Build history of the part. All positions in model axes, mm. Face numbers are marked on the shaded views. A direction names the side the tool comes from. Give positions to 0.01 mm unless a question says otherwise; leave off trailing zeros. Order: outer loops, then holes, each group sorted by start corner. A loop starts at its lowest first (then second) coordinate and runs counter-clockwise, first axis right, second up. Notation, with made-up numbers: M 56,74 L 80,74 A25 ccw 80,103 Z; hole C 67.25,21 d10. An arc over 180 degrees is marked long. Answer as CSV lines item,"result".
from build123d import *
from OCP.BRepFilletAPI import BRepFilletAPI_MakeChamfer

# Parameters (mm, degrees)
ODGI_CIE_BAZOWE1_DEPTH     = 200
SZKIC25_W                  = 265
SZKIC25_H                  = 70
WYTNIJ_WYCI_GNI_CIE2_DEPTH = 94
SFAZOWANIE1_SIZE           = 6
SFAZOWANIE1_SIZE2          = 10.392304845
ZAOKR_GLENIE1_R            = 10
OTW_R_POD_RUB_M51_D        = 5.5
OTW_R_POD_RUB_M51_DEPTH    = 3
OTW_R_POD_RUB_M61_D        = 6.6
OTW_R_POD_RUB_M61_DEPTH    = 3
OTW_R_POD_RUB_M52_D        = 5.5
OTW_R_POD_RUB_M62_D        = 6.6
OTW_R_POD_RUB_M62_DEPTH    = 10
OTW_R_POD_RUB_M62_TIP      = 1.982840043
WYTNIJ_WYCI_GNI_CIE3_REACH = 281.957
SZKIC48_R                  = 7
WYTNIJ_WYCI_GNI_CIE4_DEPTH = 10


# Sheet-metal steps are written as plain solids
with BuildPart() as part:
    # Szkic1 → Odgięcie bazowe1 (new, symmetric)
    with BuildSketch(Plane(origin=(0, 0, 0), x_dir=(0, 0, -1), z_dir=(1, 0, 0))):
        with BuildLine():
            Line((-60, 135), (-60, 4))
            ThreePointArc((-60, 4), (-58.828427125, 1.171572875), (-56, 0))
            Line((-56, 0), (56, 0))
            ThreePointArc((56, 0), (58.828427125, 1.171572875), (60, 4))
            Line((60, 4), (60, 150))
            Line((60, 150), (63, 150))
            Line((63, 150), (63, 4))
            ThreePointArc((63, 4), (60.949747468, -0.949747468), (56, -3))
            Line((56, -3), (-56, -3))
            ThreePointArc((-56, -3), (-60.949747468, -0.949747468), (-63, 4))
            Line((-63, 4), (-63, 135))
            Line((-63, 135), (-60, 135))
        make_face()
    extrude(amount=ODGI_CIE_BAZOWE1_DEPTH, both=True)

    # Szkic25 → Wytnij-wyciągnięcie2 (cut)
    with BuildSketch(Plane.XY.offset(63)):
        with Locations((-67.5, 32)):
            Rectangle(SZKIC25_W, SZKIC25_H)
    extrude(amount=-WYTNIJ_WYCI_GNI_CIE2_DEPTH, mode=Mode.SUBTRACT)

    # Sfazowanie1: one chamfer whose edges measure the first distance from different faces: ONE call of the kernel's chamfer builder (chamfer() names one face for all edges)
    sfazowanie1_edges_1 = [part.edges().sort_by_distance(p)[0] for p in [
        (-200, 150, -61.5),
        (-200, -1.5, -31),
    ]]
    sfazowanie1_side_1 = [part.faces().sort_by_distance(p)[0] for p in [
        (-200, -1.436894117, -43.5),
    ]]
    sfazowanie1_edges_2 = [part.edges().sort_by_distance(p)[0] for p in [
        (-200, 135, 61.5),
        (-200, 67, 61.5),
    ]]
    sfazowanie1_side_2 = [part.faces().sort_by_distance(p)[0] for p in [
        (-200, 101, 61.5),
    ]]
    sfazowanie1_edges_3 = [part.edges().sort_by_distance(p)[0] for p in [
        (200, 150, -61.5),
        (200, 135, 61.5),
    ]]
    sfazowanie1_side_3 = [part.faces().sort_by_distance(p)[0] for p in [
        (200, 0.451769567, 59.548230433),
    ]]
    sfazowanie1 = BRepFilletAPI_MakeChamfer(part.part.solid().wrapped)
    for e in sfazowanie1_edges_1:
        sfazowanie1.Add(SFAZOWANIE1_SIZE, SFAZOWANIE1_SIZE2, e.wrapped, sfazowanie1_side_1[0].wrapped)  # the first distance lies on this face
    for e in sfazowanie1_edges_2:
        sfazowanie1.Add(SFAZOWANIE1_SIZE, SFAZOWANIE1_SIZE2, e.wrapped, sfazowanie1_side_2[0].wrapped)  # the first distance lies on this face
    for e in sfazowanie1_edges_3:
        sfazowanie1.Add(SFAZOWANIE1_SIZE, SFAZOWANIE1_SIZE2, e.wrapped, sfazowanie1_side_3[0].wrapped)  # the first distance lies on this face
    add(Compound.cast(sfazowanie1.Shape()), mode=Mode.REPLACE)

    # Zaokrąglenie1
    zaokr_glenie1_edges = [part.edges().sort_by_distance(p)[0] for p in [
        (65, -1.5, -31),
        (65, 67, 61.5),
    ]]
    fillet(zaokr_glenie1_edges, radius=ZAOKR_GLENIE1_R)

    # Otwór pod śrubę M51
    with Locations(Plane.XY.offset(63)):
        with Locations((144, 79), (116, 79), (144, 51), (116, 51), (130, 65)):
            Hole(OTW_R_POD_RUB_M51_D / 2, depth=OTW_R_POD_RUB_M51_DEPTH)

    # Otwór pod śrubę M61
    with Locations(Plane(origin=(0, 0, -63), x_dir=(-1, 0, 0), z_dir=(0, 0, -1))):
        with Locations((-70, 84.5), (-70, 45.5), (50, 84.5), (50, 45.5), (170, 84.5), (170, 45.5)):
            Hole(OTW_R_POD_RUB_M61_D / 2, depth=OTW_R_POD_RUB_M61_DEPTH)

    # Otwór pod śrubę M52 (through all)
    with Locations(Plane(origin=(0, 0, -63), x_dir=(-1, 0, 0), z_dir=(0, 0, -1))):
        with Locations((-172.5, 125), (-57.5, 125), (57.5, 125), (172.5, 125)):
            Hole(OTW_R_POD_RUB_M52_D / 2)

    # Otwór pod śrubę M62
    with Locations(Plane(origin=(0, -3, 0), x_dir=(-1, 0, 0), z_dir=(0, -1, 0))):
        with Locations((-190, 47.25), (-80, 47.25), (-151, 39.85), (-119, 39.85), (-190, -47.25), (-151, -39.85), (-119, -39.85), (-80, -47.25)):
            Hole(OTW_R_POD_RUB_M62_D / 2, depth=OTW_R_POD_RUB_M62_DEPTH)
            with Locations((0, 0, -(OTW_R_POD_RUB_M62_DEPTH + OTW_R_POD_RUB_M62_TIP / 2))):  # 118° drill point
                Cone(0, OTW_R_POD_RUB_M62_D / 2, OTW_R_POD_RUB_M62_TIP, mode=Mode.SUBTRACT)

    # Szkic43 → Wytnij-wyciągnięcie3 (cut, up to next)
    with BuildSketch(Plane(origin=(0, 0, -63), x_dir=(-1, 0, 0), z_dir=(0, 0, -1)), mode=Mode.PRIVATE) as wytnij_wyci_gni_cie3_sk1:
        with BuildLine():
            Line((130, 146), (180, 146))
            ThreePointArc((180, 146), (182, 144), (180, 142))
            Line((180, 142), (130, 142))
            ThreePointArc((130, 142), (128, 144), (130, 146))
        make_face()
    wytnij_wyci_gni_cie3_tool1 = extrude(wytnij_wyci_gni_cie3_sk1.sketch, amount=-WYTNIJ_WYCI_GNI_CIE3_REACH, mode=Mode.PRIVATE) & part.part
    # Szkic43 → Wytnij-wyciągnięcie3 (cut, up to next)
    with BuildSketch(Plane(origin=(0, 0, -63), x_dir=(-1, 0, 0), z_dir=(0, 0, -1)), mode=Mode.PRIVATE) as wytnij_wyci_gni_cie3_sk2:
        with BuildLine():
            Line((70, 146), (120, 146))
            ThreePointArc((120, 146), (122, 144), (120, 142))
            Line((120, 142), (70, 142))
            ThreePointArc((70, 142), (68, 144), (70, 146))
        make_face()
    wytnij_wyci_gni_cie3_tool2 = extrude(wytnij_wyci_gni_cie3_sk2.sketch, amount=-WYTNIJ_WYCI_GNI_CIE3_REACH, mode=Mode.PRIVATE) & part.part
    # Szkic43 → Wytnij-wyciągnięcie3 (cut, up to next)
    with BuildSketch(Plane(origin=(0, 0, -63), x_dir=(-1, 0, 0), z_dir=(0, 0, -1)), mode=Mode.PRIVATE) as wytnij_wyci_gni_cie3_sk3:
        with BuildLine():
            Line((10, 146), (60, 146))
            ThreePointArc((60, 146), (62, 144), (60, 142))
            Line((60, 142), (10, 142))
            ThreePointArc((10, 142), (8, 144), (10, 146))
        make_face()
    wytnij_wyci_gni_cie3_tool3 = extrude(wytnij_wyci_gni_cie3_sk3.sketch, amount=-WYTNIJ_WYCI_GNI_CIE3_REACH, mode=Mode.PRIVATE) & part.part
    add(wytnij_wyci_gni_cie3_tool1.solids().sort_by_distance((-155, 144, -63))[0], mode=Mode.SUBTRACT)
    add(wytnij_wyci_gni_cie3_tool2.solids().sort_by_distance((-95, 144, -63))[0], mode=Mode.SUBTRACT)
    add(wytnij_wyci_gni_cie3_tool3.solids().sort_by_distance((-35, 144, -63))[0], mode=Mode.SUBTRACT)

    # Szkic48 → Wytnij-wyciągnięcie4 (cut)
    with BuildSketch(Plane.XY.offset(63)):
        with Locations((130, 65)):
            Circle(SZKIC48_R)
    extrude(amount=-WYTNIJ_WYCI_GNI_CIE4_DEPTH, mode=Mode.SUBTRACT)


solid = part.part
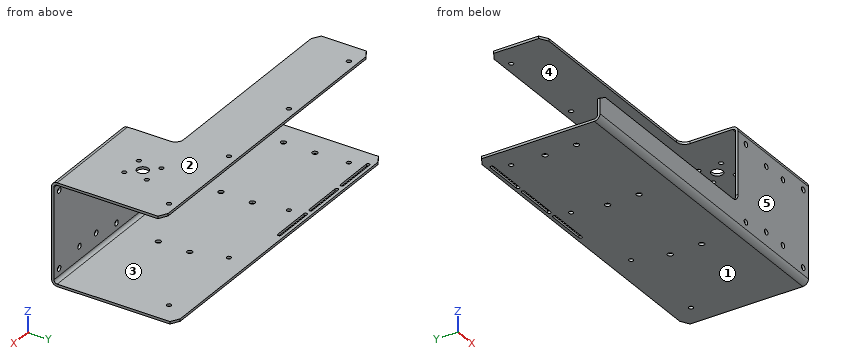
Item 1: Band-saw the part on A-A (x = -139). Give the cut face in (y, z), and give its area (3 significant figures).
Geometry says:
outline,"M -3,-56 A7 ccw 4,-63 L 142,-63 L 142,-60 L 4,-60 A4 cw 0,-56 L 0,-31 L -3,-31 Z; M 67,60 L 135,60 L 135,63 L 67,63 Z; M 146,-63 L 150,-63 L 150,-60 L 146,-60 Z"
area,"731 mm2"
Item 2: Probe line 1 along X through (y, z) = (-1, -47); line 2 along X through (y, z) = (84, -62); line 3 along Y through (x, z) = (70, -61.8). List the from-to ranges inside material, lowest first. Write a range as from..to.
Geometry says:
line 1,"x = -200..76.71, 83.29..186.71, 193.29..200"
line 2,"x = -200..-173.26, -166.74..-53.26, -46.74..66.74, 73.26..200"
line 3,"y = 0.08..42.2, 48.8..81.2, 87.8..150"
Item 3: Drop flat-ended pins along their axis: pin 1 (4.5 mm diameter, centred on x = -57.5, y = 125, fed in from -Z); pin 2 (3.5 mm diameter, centred on x = -143.5, z = -62, fed in from -Y); pin 3 (1.5 mm diameter, centred on x = -80.5, y = -1.5, fed in from +Z); pin 4 (6 mm diameter, centred on x = -170, y = 84.5, fed in from -Z). Give the stop position or say it passes through.
Geometry says:
pin 1,"passes through"
pin 2,"stops at y = -1.56"
pin 3,"stops at z = -31"
pin 4,"stops at z = 60"
Item 4: Band-saw the part on C-C (x = 45.5). Give the cut face in (y, z), and give its area (3 significant figures).
Geometry says:
outline,"M -3,-56 A7 ccw 4,-63 L 150,-63 L 150,-60 L 4,-60 A4 cw 0,-56 L 0,-31 L -3,-31 Z; M 67,60 L 135,60 L 135,63 L 67,63 Z"
area,"743 mm2"
Item 5: Pull direction Z, two halves, no side cores. Call the marked faces 1, 2 and 3: released by +Z, released by -Z, zero draft, split by the parting line, or undercut.
Geometry says:
face 1,"released by -Z"
face 2,"released by +Z"
face 3,"undercut"
Item 6: Band-saw the part on B-B (y = 25). Give the cut face in (x, z), and give its area (4 significant figures).
Geometry says:
outline,"M -200,-63 L 200,-63 L 200,-60 L -200,-60 Z; M 65,60 L 200,60 L 200,63 L 65,63 Z"
area,"1,605 mm2"
Item 7: Band-saw the part on D-D (z = -13). Give the cut face in (x, y).
Geometry says:
outline,"M 65,-3 L 200,-3 L 200,0 L 65,0 Z"
Item 8: 3-axis set-ups, long thin cutter, end or side, ignore diameter. For the marked faces 4 and 5: which of +Z, -Z, +X, -X, +Y, -Y reach the whole face in a straight line?
Geometry says:
face 4,"+X, -X, +Y"
face 5,"+Z, -Z, +X, -X, -Y"
